Autodesk Inventor part; units mm, degrees
ref_plane "YZ Plane" through (0, 0, 0) normal (1, 0, 0) x (0, 1, 0)
ref_plane "XZ Plane" through (0, 0, 0) normal (0, 1, 0) x (-1, 0, 0)
ref_plane "XY Plane" through (0, 0, 0) normal (0, 0, 1) x (1, 0, 0)
sketch "スケッチ1" plane through (0, 0, 0) normal (0, 0, 1) x (1, 0, 0)
  circle A0 centre (0, 0) radius 10
  circle A1 centre (0, 0) radius 52 construction
  line L0 (30, 30) -> (-30, 30) construction
  line L1 (-30, 30) -> (-30, -30) construction
  line L2 (-30, -30) -> (30, -30) construction
  line L3 (30, -30) -> (30, 30) construction
  line L4 (30, 30) -> (-30, -30) construction
  line L5 (-30, 30) -> (30, -30) construction
  circle A2 centre (-30, 30) radius 1.6
  circle A3 centre (-30, 0) radius 1.6
  circle A4 centre (-30, -30) radius 1.6
  circle A5 centre (30, 30) radius 1.6
  circle A6 centre (30, 0) radius 1.6
  circle A7 centre (30, -30) radius 1.6
  circle A8 centre (-28.6115, 82.3636) radius 23.5 construction
  circle A9 centre (0, 0) radius 57 construction
  circle A10 centre (-28.6115, 82.3636) radius 10
  circle A11 centre (0, 300) radius 10
  line L6 (0, 300) -> (-28.6115, 82.3636) construction
  line L7 (-5, 89.3456) -> (-49.6161, 95.211) construction
  line L8 (-49.6161, 95.211) -> (-52.223, 75.3817) construction
  line L9 (-52.223, 75.3817) -> (-7.6069, 69.5162) construction
  line L10 (-7.6069, 69.5162) -> (-5, 89.3456) construction
  line L11 (-5, 89.3456) -> (-52.223, 75.3817) construction
  line L12 (-49.6161, 95.211) -> (-7.6069, 69.5162) construction
  line L13 (-6.1752, 99.5861) -> (-45.834, 104.7999) construction
  line L14 (-45.834, 104.7999) -> (-51.0477, 65.1411) construction
  line L15 (-51.0477, 65.1411) -> (-11.389, 59.9274) construction
  line L16 (-11.389, 59.9274) -> (-6.1752, 99.5861) construction
  line L17 (-6.1752, 99.5861) -> (-51.0477, 65.1411) construction
  line L18 (-45.834, 104.7999) -> (-11.389, 59.9274) construction
  circle A12 centre (-45.834, 104.7999) radius 1.25
  circle A13 centre (-49.6161, 95.211) radius 1.25
  circle A14 centre (-52.223, 75.3817) radius 1.25
  circle A15 centre (-51.0477, 65.1411) radius 1.25
  circle A16 centre (-6.1752, 99.5861) radius 1.25
  circle A17 centre (-5, 89.3456) radius 1.25
  circle A18 centre (-7.6069, 69.5162) radius 1.25
  circle A19 centre (-11.389, 59.9274) radius 1.25
  circle A20 centre (-5, 89.3456) radius 5 construction
  circle A21 centre (-7.6069, 69.5162) radius 4 construction
  line L19 (0, 0) -> (0, 174.5579) construction
  circle A22 centre (28.6115, 82.3636) radius 23.5
  circle A23 centre (-11.389, 59.9274) radius 4 construction
  arc A24 (0, 320) -> (-19.7236, 303.3137) centre (0, 300) ccw
  arc A25 (-54.547, 96.0395) -> (-54.5734, 95.8628) centre (-49.6161, 95.211) ccw
  arc A26 (-57.1803, 76.0334) -> (-57.1904, 74.8116) centre (-52.223, 75.3817) ccw
  arc A27 (-56.0151, 64.571) -> (-55.3611, 62.6124) centre (-51.0477, 65.1411) ccw
  arc A28 (-34.9775, -29.5267) -> (-30, -35) centre (-30, -30) ccw
  line L20 (-54.5734, 95.8628) -> (-57.1803, 76.0334)
  line L21 (-57.1904, 74.8116) -> (-56.0151, 64.571)
  arc A29 (-34.9775, -29.5267) -> (-55.3611, 62.6124) centre (-187.7511, -15) ccw
  arc A30 (-31.6722, 4.7121) -> (-34.6924, -1.7267) centre (-30, 0) ccw construction
  line L22 (-19.7236, 303.3137) -> (-54.547, 96.0395)
  line L23 (-30, -35) -> (0, -35)
  circle A31 centre (-23.9585, 260) radius 1.6
  circle A32 centre (-43.8406, 141.6585) radius 1.6
  line L24 (-23.9585, 260) -> (-43.8406, 141.6585) construction
  circle A33 centre (-33.8996, 200.8293) radius 1.6
  arc A34 (19.7236, 303.3137) -> (0, 320) centre (0, 300) ccw
  arc A35 (54.5734, 95.8628) -> (54.547, 96.0395) centre (49.6161, 95.211) ccw
  arc A36 (57.1904, 74.8116) -> (57.1803, 76.0334) centre (52.223, 75.3817) ccw
  arc A37 (55.3611, 62.6124) -> (56.0151, 64.571) centre (51.0477, 65.1411) ccw
  arc A38 (30, -35) -> (34.9775, -29.5267) centre (30, -30) ccw
  line L25 (54.5734, 95.8628) -> (57.1803, 76.0334)
  line L26 (57.1904, 74.8116) -> (56.0151, 64.571)
  arc A39 (55.3611, 62.6124) -> (34.9775, -29.5267) centre (187.7511, -15) ccw
  line L27 (19.7236, 303.3137) -> (54.547, 96.0395)
  line L28 (30, -35) -> (0, -35)
  circle A40 centre (23.9585, 260) radius 1.6
  circle A41 centre (43.8406, 141.6585) radius 1.6
  circle A42 centre (33.8996, 200.8293) radius 1.6
  dimension "d0" = 20
  dimension "d1" = 104
  dimension "d2" = 60
  dimension "d3" = 60
  dimension "d4" = 3.2
  dimension "d5" = 3.2
  dimension "d6" = 3.2
  dimension "d7" = 3.2
  dimension "d8" = 3.2
  dimension "d9" = 3.2
  dimension "d10" = 47
  dimension "d12" = 5
  dimension "d13" = 20
  dimension "d14" = 20
  dimension "d15" = 300
  dimension "d16" = 20
  dimension "d17" = 45
  dimension "d18" = 40
  dimension "d19" = 40
  dimension "d20" = 2.5
  dimension "d21" = 2.5
  dimension "d22" = 2.5
  dimension "d23" = 2.5
  dimension "d24" = 2.5
  dimension "d25" = 2.5
  dimension "d26" = 2.5
  dimension "d27" = 2.5
  dimension "d28" = 10
  dimension "d29" = 8
  dimension "d30" = 8
  dimension "d31" = 20
  dimension "d33" = 5
  dimension "d34" = 5
  dimension "d35" = 5
  dimension "d36" = 5
  dimension "d37" = 5
  dimension "d38" = 3.2
  dimension "d39" = 3.2
  dimension "d40" = 3
  dimension "d41" = 120
  dimension "d42" = 40
  dimension "d43" = 3.2
extrude "押し出し1" add sketch "スケッチ1" along normal blind 4
properties part number "関節3_側板1" material "アルミニウム 6061"
Here's how the part is built. I have some questions about the finished solid (model axes, mm). Coordinates: 2 decimals unless noted, no trailing zeros. Loops run counter-clockwise (first coordinate to the right, second up) from the corner with the lowest first, then second, coordinate; pieces in that order, holes last. Notation, with made-up numbers: (10.25, -2) -> (38.25, -2) arc R26 cw to (38.25, 27) -> close; hole circle Ø3 at (38.5, 36). An arc over 180 degrees is marked (long way). Use one line per item in the form item = value. Start each with the question number.
(1) If we section it at A-A (y = 300): Please give me the cut outline in (x, z), then the cut area to 3 significant figures.
(2) If we section it at D-D (y = 134.5): Please give me the cut outline in (x, z).
(3) Will these pins go through, and if not, where does the flat tip stop? pin 1 (18 mm diameter, centred on x = -28.61, y = 82.36, fed in from +Z); pin 2 (1.5 mm diameter, centred on y = 140.5, z = 2, fed in from +X); pin 3 (1 mm diameter, centred on y = 34.5, z = 1.5, fed in from -X).
(4) We'd pull the mould along X, two halves only. Please class faces 1 (the face through (-1, 145, 4)), 2 (the face through (9.96, 96.66, 1.97)), 3 (the face through (-38.058, 18.804, 1.972)): pulls with the +X half, pulls with the -X half, needs draft (parallel to the pull), parting line crosses it, or undercut.
(5) If we section it at B-B (y = 219.5): Please give me the cut outline in (x, z), then the cut area to 3 significant figures.
(6) If we section it at C-C (z = 0.8): Give the number of separate pieces and of enclosed holes in the cut face, then the cut area to 3 significant figures.
(7) Please list where these lines run through material, in increasing order: line 1 along Y through (x, z) = (-6.5, 3.85); line 2 along Y through (x, z) = (15, 3.45); line 3 along X through (y, z) = (212, 3.3).
Verdict:
q1.outline = (-20.28, 0) -> (-10, 0) -> (-10, 4) -> (-20.28, 4) -> close; (10, 0) -> (20.28, 0) -> (20.28, 4) -> (10, 4) -> close
q1.area = 82.2 mm²
q2.outline = (-48.09, 0) -> (48.09, 0) -> (48.09, 4) -> (-48.09, 4) -> close
q3.pin_1 = through
q3.pin_2 = 47.2
q3.pin_3 = -42.66
q4.face_1 = needs draft
q4.face_2 = undercut
q4.face_3 = pulls with the -X half
q5.outline = (-33.8, 0) -> (33.8, 0) -> (33.8, 4) -> (-33.8, 4) -> close
q5.area = 270 mm²
q6.separate_pieces = 1
q6.enclosed_holes = 24
q6.area = 24,600 mm²
q7.line_1 = -35 to -7.6, 7.6 to 68.94, 70.1 to 98.38, 100.79 to 292.4, 307.6 to 318.91
q7.line_2 = -35 to 63.21, 101.52 to 313.23
q7.line_3 = -35.06 to 35.06
